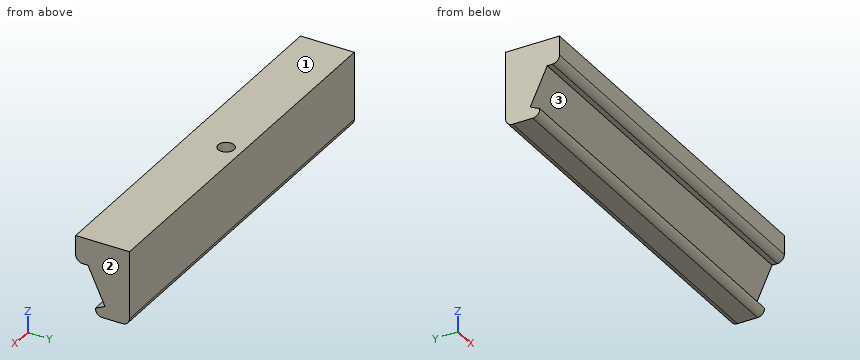
from build123d import *

# Parameters (mm, degrees)
PROFILEBOSS_EXTRUDE1_DEPTH      = 110
SKETCH3_R                       = 2.3
MOUNTINGHOLESCUT_EXTRUDE3_DEPTH = 4.5


with BuildPart() as part:
    # Sketch1 → ProfileBoss-Extrude1 (new body)
    with BuildSketch(Plane(origin=(0, 0, 0), x_dir=(0, 0, -1), z_dir=(1, 0, 0))):
        with BuildLine():
            Line((0, 0), (5.499461553, 0))
            ThreePointArc((5.499461553, 0), (6.914055855, 0.585944145), (7.5, 2.000538447))
            Line((7.5, 2.000538447), (7.5, 3.5))
            Line((7.5, 3.5), (17.922539551, 8.36011001))
            Line((17.922539551, 8.36011001), (19.190394336, 5.641186649))
            ThreePointArc((19.190394336, 5.641186649), (20.700753359, 6.16912635), (21.340729536, 7.635528477))
            Line((21.340729536, 7.635528477), (21.340729536, 13.36011001))
            ThreePointArc((21.340729536, 13.36011001), (20.754943098, 14.774323572), (19.340729536, 15.36011001))
            Line((19.340729536, 15.36011001), (0, 15.36011001))
            Line((0, 15.36011001), (0, 0))
        make_face()
    extrude(amount=PROFILEBOSS_EXTRUDE1_DEPTH)

    # Sketch3 → MountingHolesCut-Extrude3 (cut)
    with BuildSketch(Plane.XY):
        with Locations((55, 10.86011001)):
            Circle(SKETCH3_R)
    extrude(amount=-MOUNTINGHOLESCUT_EXTRUDE3_DEPTH, mode=Mode.SUBTRACT)


solid = part.part
The listing builds one solid part. Answer for the finished solid, in the listing's coordinates (mm). Face numbers are marked on the shaded views. Round coordinates to 2 decimals unless told otherwise and drop trailing zeros. Write each loop counter-clockwise with the first axis right and the second up, starting at its lowest first coordinate (ties: lowest second). Pieces come first, ordered by that corner, then holes. Notation, with made-up numbers: (83.25, 40.25) - (108.25, 40.25) arc R24 cw to (108.25, 63.25) - close; hole circle Ø5 at (-17, 5). An arc over 180 degrees is marked (long way). Use one line per item in the form item = value. Start each with the question number.
Item 1: Determine the mould class of the marked faces 1, 2 and 3 for opening direction Z: +Z half, -Z half, draft (parallel to the pull), parting line (faces both ways), or undercut.
Item 2: A cutting plane is placed at A-A (x = 63.5). Write down the section's boundary in (y, z).
Item 3: Find the intervals of material crossed by line 1 (Y direction, x = 55, z = -2.9); line 2 (Z direction, x = 83, y = 2); line 3 (Y direction, x = 76.5, z = -13.5), in increasing order. Write a range as [from, to].
Item 4: A cutting plane is placed at B-B (z = -11.5). Write down the section's boundary in (x, y), plus the area to 3 significant figures.
Item 5: A cutting plane is placed at C-C (z = -6.5). Write down the section's boundary in (x, y), plus the area to 3 significant figures.
Item 6: Flat-ended cylindrical pins translate along their axes: pin 1 Ø1.4 at (x, y) = (55.5, 11.5) entering from +Z; pin 2 Ø1.2 at (x, y) = (54, 2.5) entering from -Z. Find the tip coordinate at first contact, or state that the pin passes through.
The answers:
q1.face_1 = +Z half
q1.face_2 = draft
q1.face_3 = undercut
q2.outline = (0, -5.5) arc R2 ccw to (2, -7.5) - (3.5, -7.5) - (8.36, -17.92) - (5.64, -19.19) arc R2 ccw to (7.64, -21.34) - (13.36, -21.34) arc R2 ccw to (15.36, -19.34) - (15.36, 0) - (0, 0) - close
q3.line_1 = [0, 8.56], [13.16, 15.36]
q3.line_2 = [-7.5, 0]
q3.line_3 = [6.3, 15.36]
q4.outline = (0, 5.37) - (110, 5.37) - (110, 15.36) - (0, 15.36) - close
q4.area = 1,100 mm^2
q5.outline = (0, 0.27) - (110, 0.27) - (110, 15.36) - (0, 15.36) - close
q5.area = 1,660 mm^2
q6.pin_1 = -4.5
q6.pin_2 = -7.5
